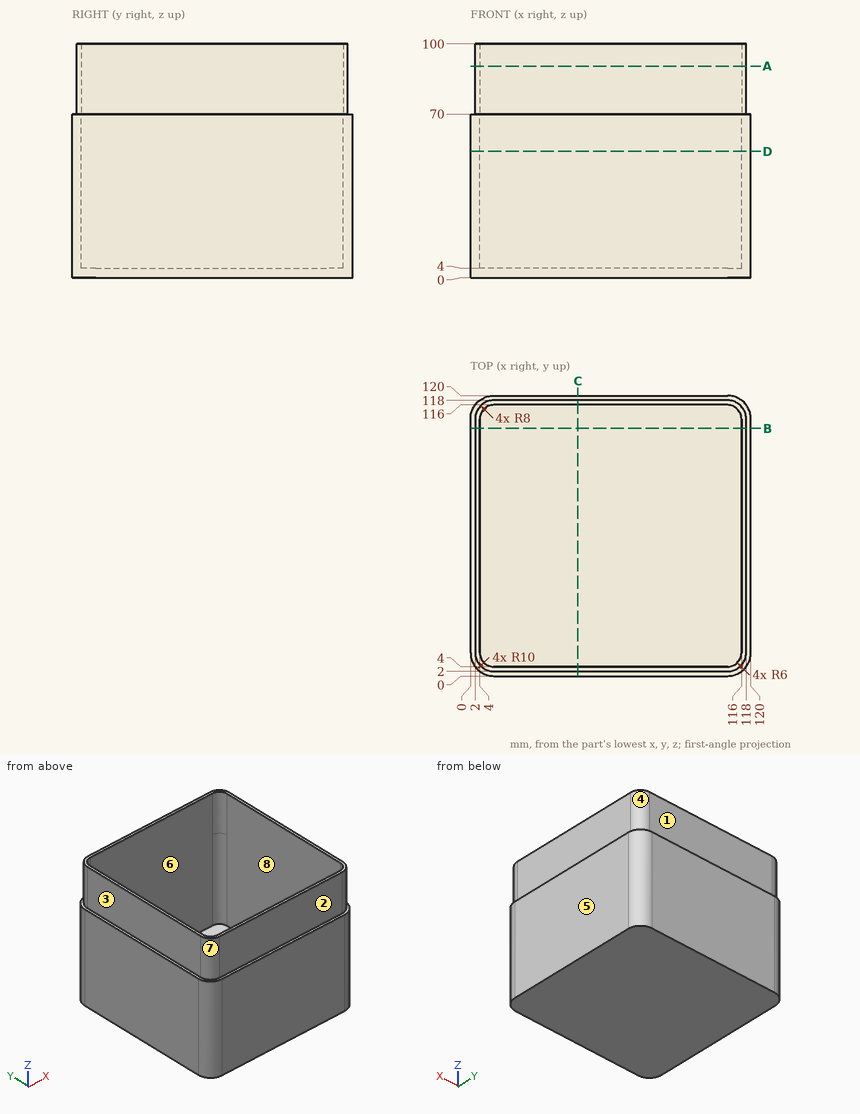
The drawing under review shows one solid part. Ordinate dimensions are in mm from its lowest x, y, z. A direction names the side the tool comes from. Coordinates: 2 decimals unless noted, no trailing zeros. Order: outer loops, then holes, each group sorted by start corner. A loop starts at its lowest first (then second) coordinate and runs counter-clockwise, first axis right, second up. Notation, with made-up numbers: (-26, 34.5) -> (26, 34.5) arc R16 cw to (26, 41.5) -> close; hole circle Ø7 at (-25.75, -39.5). An arc over 180 degrees is marked (long way). Answer as CSV lines item,"result".
Q1. We need section A-A (z = 90.5). State the section outline as (x, y) points, plus the area to 3 significant figures.
Model answer:
outline,"(2, 10) arc R8 ccw to (10, 2) -> (110, 2) arc R8 ccw to (118, 10) -> (118, 110) arc R8 ccw to (110, 118) -> (10, 118) arc R8 ccw to (2, 110) -> close; hole (4, 10) arc R6 ccw to (10, 4) -> (110, 4) arc R6 ccw to (116, 10) -> (116, 110) arc R6 ccw to (110, 116) -> (10, 116) arc R6 ccw to (4, 110) -> close"
area,"888 mm2"
Q2. Clearance check with flat-ended pins moving along their axes: pin 1 Ø24 at (y, z) = (78.5, 92) entering from +X; pin 2 Ø3 at (x, y) = (101, 104.5) entering from +Z; pin 3 Ø15 at (x, z) = (72, 88.5) entering from +Y. State where each tip first meets the part, or that it passes through.
Model answer:
pin 1,"stops at x = 118"
pin 2,"stops at z = 4"
pin 3,"stops at y = 118"
Q3. We need section D-D (z = 54). State the section outline as (x, y) points, plus the area to 3 significant figures.
Model answer:
outline,"(0, 10) arc R10 ccw to (10, 0) -> (110, 0) arc R10 ccw to (120, 10) -> (120, 110) arc R10 ccw to (110, 120) -> (10, 120) arc R10 ccw to (0, 110) -> close; hole (4, 10) arc R6 ccw to (10, 4) -> (110, 4) arc R6 ccw to (116, 10) -> (116, 110) arc R6 ccw to (110, 116) -> (10, 116) arc R6 ccw to (4, 110) -> close"
area,"1,800 mm2"
Q4. For the marked faces 1, 2, 3 and 4, list the 3-axis set-ups (+Z, -Z, +X, -X, +Y, -Y) from which the entire face can be reached by the end or side of a thin tool; tool diameter is ignored.
Model answer:
face 1,"+Z, +X, -X, +Y"
face 2,"+Z, +X, -X, -Y"
face 3,"+Z, -X, +Y, -Y"
face 4,"+Z, +X, +Y"
Q5. Draft analysis for pull direction X (two halves, no side actions). For the marked faces 5, 6, 7 and 8, state which applies: released by +X, released by -X, zero draft, split by the parting line, or undercut.
Model answer:
face 5,"released by +X"
face 6,"undercut"
face 7,"released by -X"
face 8,"undercut"
Q6. We need section B-B (y = 106). State the section outline as (x, z) points.
Model answer:
outline,"(0, 0) -> (120, 0) -> (120, 70) -> (118, 70) -> (118, 100) -> (116, 100) -> (116, 4) -> (4, 4) -> (4, 100) -> (2, 100) -> (2, 70) -> (0, 70) -> close"
Q7. Wall thickness on line 1 along Y through (x, z) = (20, 16); line 2 along Y through (x, z) = (101, 78.5): over which ranges is each line inside the solid? List them lowest first. Write a range as [from, to].
Model answer:
line 1,"y = [0, 4], [116, 120]"
line 2,"y = [2, 4], [116, 118]"
